Geometry check sheet. Reference: the model listing, model coordinates, mm. Coordinates: 2 decimals unless noted, no trailing zeros. Write each loop counter-clockwise with the first axis right and the second up, starting at its lowest first coordinate (ties: lowest second). Pieces come first, ordered by that corner, then holes. Notation, with made-up numbers: (68.5, 45) - (121.5, 45) arc R33 cw to (121.5, 81) - close; hole circle Ø11 at (89, 17.5). An arc over 180 degrees is marked (long way). Answer as a JSON object with one key per item and string values. Group by question number.
Autodesk Inventor part; units mm, degrees
sketch "Эскиз1" plane through (0, 0, 0) normal (1, 0, 0) x (0, 1, 0)
  line L0 (-146.2, 57.5) -> (127.8, 57.5)
  line L1 (138.3, 47) -> (138.3, -47)
  line L2 (127.8, -57.5) -> (-146.2, -57.5)
  line L3 (-156.7, -47) -> (-156.7, 47)
  line L4 (-227.1367, 0) -> (250.6977, 0)
  arc A0 (-146.2, 57.5) -> (-156.7, 47) centre (-146.2, 47) ccw
  arc A1 (-156.7, -47) -> (-146.2, -57.5) centre (-146.2, -47) ccw
  arc A2 (127.8, -57.5) -> (138.3, -47) centre (127.8, -47) ccw
  arc A3 (138.3, 47) -> (127.8, 57.5) centre (127.8, 47) ccw
  line L5 (-66.5644, 51) -> (182.4356, 51)
  line L6 (131.8, 34) -> (131.8, -35)
  line L7 (182.4356, -51) -> (-66.5644, -51)
  line L8 (-150.2, -35) -> (-150.2, 34)
  circle A4 centre (-79.7, 51) radius 3
  circle A5 centre (-9.2, 51) radius 3
  circle A6 centre (61.3, 51) radius 3
  circle A7 centre (-79.7, -51) radius 3
  circle A8 centre (-9.2, -51) radius 3
  circle A9 centre (61.3, -51) radius 3
  circle A10 centre (131.8, -0.5) radius 3
  circle A11 centre (-150.2, -0.5) radius 3
  line L9 (-150.2, 34) -> (-150.2, 51)
  line L10 (-150.2, 51) -> (-66.5644, 51)
  line L11 (182.4356, 51) -> (131.8, 51)
  line L12 (131.8, 51) -> (131.8, 34)
  line L13 (131.8, -35) -> (131.8, -51)
  line L14 (131.8, -51) -> (181.2224, -51)
  line L15 (-66.5644, -51) -> (-150.2, -51)
  line L16 (-150.2, -36.3739) -> (-150.2, -51)
  circle A12 centre (-150.2, 51) radius 3
  circle A13 centre (-150.2, -51) radius 3
  circle A14 centre (131.8, -51) radius 3
  circle A15 centre (131.8, 51) radius 3
  line L17 (0, -83.5445) -> (0, 83.5445)
  point P0 (0, 0)
  dimension "d0" = 115
  dimension "d1" = 295
  dimension "d2" = 10.5
  dimension "d3" = 10.5
  dimension "d7" = 6.5
  dimension "d8" = 6.5
  dimension "d9" = 6.5
  dimension "d10" = 6.5
  dimension "d15" = 6
  dimension "d16" = 6
  dimension "d17" = 6
  dimension "d19" = 6
  dimension "d20" = 6
  dimension "d21" = 6
  dimension "d23" = 6
  dimension "d24" = 6
  dimension "d25" = 70.5
  dimension "d26" = 70.5
  dimension "d27" = 70.5
  dimension "d28" = 6
  dimension "d29" = 6
  dimension "d30" = 6
  dimension "d31" = 6
  dimension "d34" = 70.5
  dimension "d35" = 70.5
  dimension "d36" = 70.5
  dimension "d37" = 138.3
extrude "Выдавливание1" add sketch "Эскиз1" along normal blind 3.5 contours L0 L17 L5 A5 L10 A4 A12 L9 L8 A11 L4 L3 A0 | L0 A3 L5 A15 A6 L17 | L17 L4 A11 L8 L9 A12 L10 A4 L5 A5 | L5 A6 A15 L12 L6 A10 L4 L17 | A13 L16 L15 | L15 L16 A13 | A7 L15 | L15 A7 | A8 L7 | L7 A8 | L4 A11 L17 L2 A1 L3 | A3 L1 L4 A10 L6 L12 A15 L5 | A5 L5 | L5 A5 | A6 L5 | L5 A6 | L4 A10 L6 L13 A14 L7 A9 L17 | A11 L8 L4 | L4 L8 A11 | A15 L12 L5 | L5 A15 | A11 L8 L4 | L4 L8 A11 | A10 L6 L4 | L4 L6 A10 | L7 A9 A14 A2 L2 L17 | L1 A2 L7 A14 L13 L6 A10 L4 | L12 A15 L5 | L6 A10 L4 | L4 A10 L6 | A9 L7 | L7 A9 | L10 A4 | A4 L10 | A12 L10 L9 | L9 L10 A12 | A14 L7 L13 | L13 L7 A14 | L7 A14
extrude "Выдавливание2" cut sketch "Эскиз1" along normal blind 5 contours A13 L16 L15 | L15 L16 A13 | A7 L15 | L15 A7 | A8 L7 | L7 A8 | A5 L5 | L5 A5 | A6 L5 | L5 A6 | A11 L8 L4 | L4 L8 A11 | A15 L12 L5 | L5 A15 | A11 L8 L4 | L4 L8 A11 | A10 L6 L4 | L4 L6 A10 | L12 A15 L5 | L6 A10 L4 | L4 A10 L6 | A9 L7 | L7 A9 | L10 A4 | A4 L10 | A12 L10 L9 | L9 L10 A12 | A14 L7 L13 | L13 L7 A14 | L7 A14
properties part number "крыша"
(1) Section check A-A (y = -79.7). Record the cut outline in (x, z), and give its area (4 significant figures).
(2) Draft check along Y on faces 1 (the face through (1.7, -153.2, 50.9)), 2 (the face through (3.5, -11, 1)), 3 (the face through (1.73, 135.14, 54.51)), 4 (the face through (1.73, 62.91, 48.47)). Enter one of: +Y half, -Y half, draft (parallel to the pull), parting line (faces both ways), or undercut.
(3) Section check B-B (z = 51). Record the cut outline in (x, y), and give its area (3 significant figures).
(4) Material ranges on L1, parallel to Z at x = 2.55, y = -79.7; L2, parallel to Y at x = 1.85, z = -0.5; L3, parallel to Y at x = 1.9, z = -51, recorded low to high. Write a range as [from, to].
(5) Gauge pin test, flat ends, axial feed: pin 1 (9.5 mm diameter, centred on y = -150.2, z = 51, fed in from -X); pin 2 (5 mm diameter, centred on y = -79.7, z = 51, fed in from -X). Record the tip position at first contact, or that the pin passes through.
(6) Section check C-C (y = 131.8). Record the cut outline in (x, z), and give its area (3 significant figures).
Conclusion:
{
 "1": {"outline": "(0, -57.5) - (3.5, -57.5) - (3.5, -54) - (0, -54) - close; (0, -48) - (3.5, -48) - (3.5, 48) - (0, 48) - close; (0, 54) - (3.5, 54) - (3.5, 57.5) - (0, 57.5) - close", "area": "360.5 mm^2"},
 "2": {"face 1": "undercut", "face 2": "draft", "face 3": "+Y half", "face 4": "undercut"},
 "3": {"outline": "(0, -155.91) - (3.5, -155.91) - (3.5, -153.2) - (0, -153.2) - close; (0, -147.2) - (3.5, -147.2) - (3.5, -82.7) - (0, -82.7) - close; (0, -76.7) - (3.5, -76.7) - (3.5, -12.2) - (0, -12.2) - close; (0, -6.2) - (3.5, -6.2) - (3.5, 58.3) - (0, 58.3) - close; (0, 64.3) - (3.5, 64.3) - (3.5, 128.8) - (0, 128.8) - close; (0, 134.8) - (3.5, 134.8) - (3.5, 137.51) - (0, 137.51) - close", "area": "922 mm^2"},
 "4": {"L1": "z = [-57.5, -54], [-48, 48], [54, 57.5]", "L2": "y = [-156.7, -153.2], [-147.2, 128.8], [134.8, 138.3]", "L3": "y = [-155.91, -153.2], [-147.2, -82.7], [-76.7, -12.2], [-6.2, 58.3], [64.3, 128.8], [134.8, 137.51]"},
 "5": {"pin 1": "stops at x = 0", "pin 2": "passes through"},
 "6": {"outline": "(0, -56.71) - (3.5, -56.71) - (3.5, -54) - (0, -54) - close; (0, -48) - (3.5, -48) - (3.5, -3.5) - (0, -3.5) - close; (0, 2.5) - (3.5, 2.5) - (3.5, 48) - (0, 48) - close; (0, 54) - (3.5, 54) - (3.5, 56.71) - (0, 56.71) - close", "area": "334 mm^2"}
}
